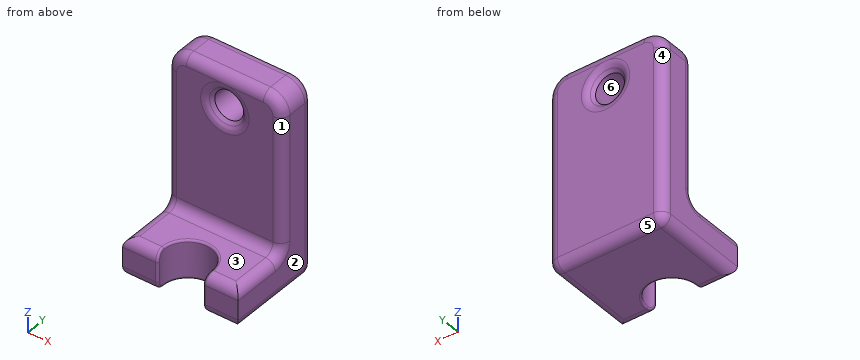
from build123d import *

# Parameters (mm, degrees)
F0_R         = 7.5
F1_DEPTH     = 20
F2_SIZE      = 3
F3_W         = 60
F3_H         = 20
F4_DEPTH     = 30
F5_T1_DEPTH  = 60
F5_T3_DEPTH  = 65
F5_T5_DEPTH  = 40
F5_T7_DEPTH  = 37.5
F5_T9_DEPTH  = 85
F5_T12_ANGLE = 90
F5_T14_ANGLE = 90
F5_T18_ANGLE = 90
F5_T20_ANGLE = 90
F6_T1_DEPTH  = 40
F6_T3_DEPTH  = 85
F6_T5_DEPTH  = 50
F6_T7_DEPTH  = 57.5
F6_T9_DEPTH  = 85
F6_S13_W     = 5
F6_S13_H     = 5
F6_T14_DEPTH = 5
F6_S19_W     = 5
F6_S19_H     = 5
F6_T20_DEPTH = 5
F6_T26_ANGLE = 90
F6_T28_ANGLE = 90
F8_DEPTH     = 20.001
F9_R         = 1


# Not quite as in the source:
# - a fillet or chamfer that OpenCascade refuses, or shapes differently, is made with other operations: its cross-section is extruded or revolved along the edge and cut away or added


with BuildPart() as f1:
    # F0 (on Front) → F1 (new body)
    with BuildSketch(Plane.XZ):
        with BuildLine():
            Line((20, 50), (-20, 50))
            ThreePointArc((-20, 50), (-27.0710678119, 47.0710678119), (-30, 40))
            Line((-30, 40), (-30, -50))
            Line((-30, -50), (30, -50))
            Line((30, -50), (30, 40))
            ThreePointArc((30, 40), (27.0710678119, 47.0710678119), (20, 50))
        make_face()
        with Locations((0, 32.5)):
            Circle(F0_R, mode=Mode.SUBTRACT)
    extrude(amount=F1_DEPTH)

    # F2
    f2_edges = [f1.edges().sort_by_distance(p)[0] for p in [
        (7.5, -10, 32.5),
        (-7.5, 0, 32.5),
        (-7.5, -20, 32.5),
    ]]
    chamfer(f2_edges, length=F2_SIZE)

    # F3 (on face) → F4 (join)
    with BuildSketch(Plane.XZ.offset(20)):
        with Locations((0, -40)):
            Rectangle(F3_W, F3_H)
    extrude(amount=F4_DEPTH)

    # F5: fillet of radius 5 on 10 edges, made by hand

    # F5_s2 → F5_t1 (join)
    with BuildSketch(Plane.YZ.offset(-30)):
        with BuildLine():
            ThreePointArc((-20, -25), (-21.4644660941, -28.5355339059), (-25, -30))
            Line((-25, -30), (-20, -30))
            Line((-20, -30), (-20, -25))
        make_face()
    extrude(amount=F5_T1_DEPTH)

    # F5_s4 → F5_t3 (cut)
    with BuildSketch(Plane.XY.offset(-25)):
        with BuildLine():
            ThreePointArc((25, -20), (28.5355339059, -18.5355339059), (30, -15))
            Line((30, -15), (30, -20))
            Line((30, -20), (25, -20))
        make_face()
        with BuildLine():
            ThreePointArc((-25, -20), (-28.5355339059, -18.5355339059), (-30, -15))
            Line((-30, -15), (-30, -20))
            Line((-30, -20), (-25, -20))
        make_face()
    extrude(amount=F5_T3_DEPTH, mode=Mode.SUBTRACT)

    # F5_s6 → F5_t5 (cut)
    with BuildSketch(Plane.YZ.offset(-20)):
        with BuildLine():
            ThreePointArc((-20, 45), (-18.5355339059, 48.5355339059), (-15, 50))
            Line((-15, 50), (-20, 50))
            Line((-20, 50), (-20, 45))
        make_face()
    extrude(amount=F5_T5_DEPTH, mode=Mode.SUBTRACT)

    # F5_s8 → F5_t7 (cut)
    with BuildSketch(Plane.XZ.offset(25)):
        with BuildLine():
            ThreePointArc((30, -35), (28.5355339059, -31.4644660941), (25, -30))
            Line((25, -30), (30, -30))
            Line((30, -30), (30, -35))
        make_face()
        with BuildLine():
            ThreePointArc((-30, -35), (-28.5355339059, -31.4644660941), (-25, -30))
            Line((-25, -30), (-30, -30))
            Line((-30, -30), (-30, -35))
        make_face()
    extrude(amount=F5_T7_DEPTH, mode=Mode.SUBTRACT)

    # F5_s10 → F5_t9 (cut)
    with BuildSketch(Plane.YZ.offset(-42.5)):
        with BuildLine():
            ThreePointArc((-45, -30), (-48.5355339059, -31.4644660941), (-50, -35))
            Line((-50, -35), (-50, -30))
            Line((-50, -30), (-45, -30))
        make_face()
    extrude(amount=F5_T9_DEPTH, mode=Mode.SUBTRACT)

    # F5_s11 → F5_t12 (revolve, cut)
    with BuildSketch(Plane.XY.offset(40)):
        with BuildLine():
            ThreePointArc((25, -20), (28.5355339059, -18.5355339059), (30, -15))
            Line((30, -15), (30, -20))
            Line((30, -20), (25, -20))
        make_face()
    revolve(axis=Axis((20, -20, 40), (0, -1, 0)), revolution_arc=F5_T12_ANGLE, mode=Mode.SUBTRACT)

    # F5_s13 → F5_t14 (revolve, cut)
    with BuildSketch(Plane.YZ.offset(-20)):
        with BuildLine():
            ThreePointArc((-20, 45), (-18.5355339059, 48.5355339059), (-15, 50))
            Line((-15, 50), (-20, 50))
            Line((-20, 50), (-20, 45))
        make_face()
    revolve(axis=Axis((-20, -20, 40), (0, -1, 0)), revolution_arc=F5_T14_ANGLE, mode=Mode.SUBTRACT)

    # F5_s15 → F5_t16 (revolve, cut)
    with BuildSketch(Plane.XY.offset(32.5)):
        with BuildLine():
            ThreePointArc((9.0355339059, -18.5355339059), (10.65765065, -19.6193976626), (12.5710678119, -20))
            Line((12.5710678119, -20), (10.5, -20))
            Line((10.5, -20), (9.0355339059, -18.5355339059))
        make_face()
    revolve(axis=Axis((0, -20, 32.5), (0, -1, 0)), mode=Mode.SUBTRACT)

    # F5_s17 → F5_t18 (revolve, cut)
    with BuildSketch(Plane.XY.offset(-25)):
        with BuildLine():
            ThreePointArc((-30, -15), (-28.5355339059, -18.5355339059), (-25, -20))
            Line((-25, -20), (-30, -20))
            Line((-30, -20), (-30, -15))
        make_face()
    revolve(axis=Axis((-30, -25, -25), (-1, 0, 0)), revolution_arc=F5_T18_ANGLE, mode=Mode.SUBTRACT)

    # F5_s19 → F5_t20 (revolve, cut)
    with BuildSketch(Plane.XY.offset(-25)):
        with BuildLine():
            ThreePointArc((30, -15), (28.5355339059, -18.5355339059), (25, -20))
            Line((25, -20), (30, -20))
            Line((30, -20), (30, -15))
        make_face()
    revolve(axis=Axis((30, -25, -25), (-1, 0, 0)), revolution_arc=F5_T20_ANGLE, mode=Mode.SUBTRACT)

    # F6: fillet of radius 5 on 10 edges, made by hand

    # F6_s2 → F6_t1 (cut)
    with BuildSketch(Plane.YZ.offset(-20)):
        with BuildLine():
            ThreePointArc((0, 45), (-1.4644660941, 48.5355339059), (-5, 50))
            Line((-5, 50), (0, 50))
            Line((0, 50), (0, 45))
        make_face()
    extrude(amount=F6_T1_DEPTH, mode=Mode.SUBTRACT)

    # F6_s4 → F6_t3 (cut)
    with BuildSketch(Plane.XY.offset(-45)):
        with BuildLine():
            ThreePointArc((-25, 0), (-28.5355339059, -1.4644660941), (-30, -5))
            Line((-30, -5), (-30, 0))
            Line((-30, 0), (-25, 0))
        make_face()
        with BuildLine():
            ThreePointArc((25, 0), (28.5355339059, -1.4644660941), (30, -5))
            Line((30, -5), (30, 0))
            Line((30, 0), (25, 0))
        make_face()
    extrude(amount=F6_T3_DEPTH, mode=Mode.SUBTRACT)

    # F6_s6 → F6_t5 (cut)
    with BuildSketch(Plane.YZ.offset(-25)):
        with BuildLine():
            ThreePointArc((0, -45), (-1.4644660941, -48.5355339059), (-5, -50))
            Line((-5, -50), (0, -50))
            Line((0, -50), (0, -45))
        make_face()
    extrude(amount=F6_T5_DEPTH, mode=Mode.SUBTRACT)

    # F6_s8 → F6_t7 (cut)
    with BuildSketch(Plane.XZ.offset(5)):
        with BuildLine():
            ThreePointArc((-30, -45), (-28.5355339059, -48.5355339059), (-25, -50))
            Line((-25, -50), (-30, -50))
            Line((-30, -50), (-30, -45))
        make_face()
        with BuildLine():
            ThreePointArc((25, -50), (28.5355339059, -48.5355339059), (30, -45))
            Line((30, -45), (30, -50))
            Line((30, -50), (25, -50))
        make_face()
    extrude(amount=F6_T7_DEPTH, mode=Mode.SUBTRACT)

    # F6_s10 → F6_t9 (cut)
    with BuildSketch(Plane.YZ.offset(-42.5)):
        with BuildLine():
            ThreePointArc((-45, -50), (-48.5355339059, -48.5355339059), (-50, -45))
            Line((-50, -45), (-50, -50))
            Line((-50, -50), (-45, -50))
        make_face()
    extrude(amount=F6_T9_DEPTH, mode=Mode.SUBTRACT)


with BuildPart() as f6_tool12:
    # F6_s13 → F6_t14 (new body)
    with BuildSketch(Plane.XY.offset(-45)):
        with Locations((-27.5, -2.5)):
            Rectangle(F6_S13_W, F6_S13_H)
    extrude(amount=-F6_T14_DEPTH)

    # F6_s15 → F6_t16 (revolve, cut)
    with BuildSketch(Plane(origin=(-25, -5, -45), x_dir=(0.7071067812, -0.7071067812, 0), z_dir=(0.7071067812, 0.7071067812, 0))):
        with BuildLine():
            ThreePointArc((0, -5), (5, 0), (0, 5))
            Line((0, 5), (0, -5))
        make_face()
    revolve(axis=Axis((-25, -5, -45), (0, 0, -1)), mode=Mode.SUBTRACT)


with BuildPart() as f1_1:
    add(f1.part)

    # F6_t11: cut F6_tool12
    add(f6_tool12.part, mode=Mode.SUBTRACT)


with BuildPart() as f6_tool18:
    # F6_s19 → F6_t20 (new body)
    with BuildSketch(Plane.XY.offset(-45)):
        with Locations((27.5, -2.5)):
            Rectangle(F6_S19_W, F6_S19_H)
    extrude(amount=-F6_T20_DEPTH)

    # F6_s21 → F6_t22 (revolve, cut)
    with BuildSketch(Plane(origin=(25, -5, -45), x_dir=(-0.7071067812, -0.7071067812, 0), z_dir=(0.7071067812, -0.7071067812, 0))):
        with BuildLine():
            ThreePointArc((0, -5), (5, 0), (0, 5))
            Line((0, 5), (0, -5))
        make_face()
    revolve(axis=Axis((25, -5, -45), (0, 0, -1)), mode=Mode.SUBTRACT)


with BuildPart() as f1_2:
    add(f1_1.part)

    # F6_t17: cut F6_tool18
    add(f6_tool18.part, mode=Mode.SUBTRACT)

    # F6_s23 → F6_t24 (revolve, cut)
    with BuildSketch(Plane.XY.offset(32.5)):
        with BuildLine():
            ThreePointArc((9.0355339059, -1.4644660941), (10.65765065, -0.3806023374), (12.5710678119, 0))
            Line((12.5710678119, 0), (10.5, 0))
            Line((10.5, 0), (9.0355339059, -1.4644660941))
        make_face()
    revolve(axis=Axis((0, 0, 32.5), (0, -1, 0)), mode=Mode.SUBTRACT)

    # F6_s25 → F6_t26 (revolve, cut)
    with BuildSketch(Plane.YZ.offset(-20)):
        with BuildLine():
            ThreePointArc((0, 45), (-1.4644660941, 48.5355339059), (-5, 50))
            Line((-5, 50), (0, 50))
            Line((0, 50), (0, 45))
        make_face()
    revolve(axis=Axis((-20, 0, 40), (0, -1, 0)), revolution_arc=F6_T26_ANGLE, mode=Mode.SUBTRACT)

    # F6_s27 → F6_t28 (revolve, cut)
    with BuildSketch(Plane.XY.offset(40)):
        with BuildLine():
            ThreePointArc((25, 0), (28.5355339059, -1.4644660941), (30, -5))
            Line((30, -5), (30, 0))
            Line((30, 0), (25, 0))
        make_face()
    revolve(axis=Axis((20, 0, 40), (0, -1, 0)), revolution_arc=F6_T28_ANGLE, mode=Mode.SUBTRACT)

    # F7 (on face) → F8 (cut, through all)
    with BuildSketch(Plane.XY.offset(-30)):
        with BuildLine():
            Line((-12.5, -45), (12.5, -45))
            ThreePointArc((12.5, -45), (0, -32.5), (-12.5, -45))
        make_face()
        with BuildLine():
            ThreePointArc((-12.5, -45), (0, -57.5), (12.5, -45))
            Line((12.5, -45), (-12.5, -45))
        make_face()
    extrude(amount=-F8_DEPTH, mode=Mode.SUBTRACT)

    # F9
    f9_edges = [f1_2.edges().sort_by_distance(p)[0] for p in [
        (0, -32.5, -50),
        (-11.98926, -48.536614, -48.534454),
        (-11.456439, -50, -40),
        (-11.98926, -48.536614, -31.465546),
        (0, -32.5, -30),
        (11.98926, -48.536614, -31.465546),
        (11.456439, -50, -40),
        (11.98926, -48.536614, -48.534454),
    ]]
    fillet(f9_edges, radius=F9_R)


solid = f1_2.part
Work out the finished part from the listing and answer in its coordinate system (mm). Face numbers are marked on the shaded views. A direction names the side the tool comes from. Give positions to 0.01 mm unless a question says otherwise; leave off trailing zeros. Write each loop counter-clockwise with the first axis right and the second up, starting at its lowest first coordinate (ties: lowest second). Pieces come first, ordered by that corner, then holes.
Q1. A tool of negligible diameter and unlimited length cuts with its end or side. For the marked faces 1, 2 and 3, from which of +Z, -Z, +X, -X, +Y, -Y can it reach the whole face along a straight path? Write none if from no direction.
Answer:
face 1: +Z, +X, -Y
face 2: +Z, -Z, +X, +Y, -Y
face 3: +Z, +X, -X, -Y
Q2. The part is cut by section A-A on y = -6.5. Give the vertices of the cut face in (x, z).
Answer:
outline: (-30, -45) arc R5 ccw to (-25, -50) - (25, -50) arc R5 ccw to (30, -45) - (30, 40) arc R10 ccw to (20, 50) - (-20, 50) arc R10 ccw to (-30, 40) - close; hole circle Ø15 at (0, 32.5)
Q3. The part is cut by section B-B on z = 32.5. Give the vertices of the cut face in (x, y).
Answer:
outline: (-30, -15) arc R5 ccw to (-25, -20) - (-12.57, -20) arc R5 ccw to (-9.04, -18.54) - (-7.5, -17) - (-7.5, -3) - (-9.04, -1.46) arc R5 ccw to (-12.57, 0) - (-25, 0) arc R5 ccw to (-30, -5) - close; (7.5, -17) - (9.04, -18.54) arc R5 ccw to (12.57, -20) - (25, -20) arc R5 ccw to (30, -15) - (30, -5) arc R5 ccw to (25, 0) - (12.57, 0) arc R5 ccw to (9.04, -1.46) - (7.5, -3) - close
Q4. The part is cut by section C-C on x = 0. Give the vertices of the cut face in (y, z).
Answer:
outline: (-32.5, -49) arc R1 ccw to (-31.5, -50) - (-5, -50) arc R5 ccw to (0, -45) - (0, 19.93) arc R5 ccw to (-1.46, 23.46) - (-3, 25) - (-17, 25) - (-18.54, 23.46) arc R5 ccw to (-20, 19.93) - (-20, -25) arc R5 cw to (-25, -30) - (-31.5, -30) arc R1 ccw to (-32.5, -31) - close; (-20, 45.04) arc R5 ccw to (-18.54, 41.54) - (-17, 40) - (-3, 40) - (-1.46, 41.54) arc R5 ccw to (0, 45.04) arc R5 ccw to (-5, 50) - (-15, 50) arc R5 ccw to start
Q5. The part is cut by section D-D on z = -9. Give the vertices of the cut face in (x, y), and give its area (3 significant figures).
Answer:
outline: (-30, -15) arc R5 ccw to (-25, -20) - (25, -20) arc R5 ccw to (30, -15) - (30, -5) arc R5 ccw to (25, 0) - (-25, 0) arc R5 ccw to (-30, -5) - close
area: 1,180 mm2
Q6. Given pin 1 (6 mm diameter, centred on x = -4.5, z = -1, fed in from -Y); pin 2 (3 mm diameter, centred on y = -19, z = -21, fed in from +X); pin 3 (8 mm diameter, centred on y = -21.5, z = -11, fed in from -X); pin 4 (13.5 mm diameter, centred on x = 0, z = 32.5, fed in from +Y), each flat-ended and moving along its own axis, determine where each tip first touches the part or whether it passes through.
Answer:
pin 1: stops at y = -20
pin 2: stops at x = 29.33
pin 3: stops at x = -29.33
pin 4: passes through
Q7. For a pull along X with two mould halves and no side action, classify the marked faces 4, 5 and 6 as released by +X, released by -X, zero draft, split by the parting line, or undercut.
Answer:
face 4: released by -X
face 5: zero draft
face 6: undercut
Q8. Straight lines are drawn through the part: L1, parallel to X at y = -45, z = -39; L2, parallel to Z at x = 0, y = -14; L3, parallel to X at y = -9, z = 32. For each, find the intervals that lie inside material, in ascending order.
Answer:
L1: x = -30 to -12.5, 12.5 to 30
L2: z = -50 to 25, 40 to 50
L3: x = -30 to -7.48, 7.48 to 30
